Model file for the job. Use its own axes, mm. A direction names the side the tool comes from. Coordinates: 2 decimals unless noted, no trailing zeros. Order: outer loops, then holes, each group sorted by start corner. A loop starts at its lowest first (then second) coordinate and runs counter-clockwise, first axis right, second up. Notation, with made-up numbers: (-5.5, -1) - (41.5, -1) arc R4 ccw to (41.5, 4) - close; hole circle Ø4 at (-29.5, 50). An arc over 180 degrees is marked (long way). Put each result on its own line as item: value. Start each with the question number.
```python
from build123d import *

# Parameters (mm, degrees)
ESQUISSE2_R             = 6
BOSS_EXTRU_1_DEPTH      = 6
ESQUISSE3_R             = 3
BOSS_EXTRU_2_DEPTH      = 15.5
ESQUISSE4_W             = 12
ESQUISSE4_H             = 0.5
ENL_V_MAT_EXTRU_1_DEPTH = 7.75
ESQUISSE5_R             = 1.5
ENL_V_MAT_EXTRU_2_DEPTH = 3.5
ESQUISSE6_W             = 3
ESQUISSE6_H             = 1
BOSS_EXTRU_3_DEPTH      = 4
ESQUISSE7_R             = 18.5
BOSS_EXTRU_4_DEPTH      = 10
BOSS_EXTRU_4_DEPTH_BACK = 5


with BuildPart() as part:
    # Esquisse1 → Révolution1 (revolve)
    with BuildSketch(Plane.XY):
        Polygon((0, 0), (0, 7), (7, 7), (7, 16), (37, 16), (37, 18.5), (59, 18.5), (59, 0), align=None)
    revolve(axis=Axis((0, 0, 0), (1, 0, 0)))

    # Esquisse2 → Boss.-Extru.1 (add)
    with BuildSketch(Plane(origin=(59, 0, 0), x_dir=(0, 0, -1), z_dir=(1, 0, 0))):
        with Locations((0, 7)):
            Circle(ESQUISSE2_R)
    extrude(amount=BOSS_EXTRU_1_DEPTH)

    # Esquisse3 → Boss.-Extru.2 (add)
    with BuildSketch(Plane(origin=(65, 0, 0), x_dir=(0, 0, -1), z_dir=(1, 0, 0))):
        with Locations((0, 7)):
            Circle(ESQUISSE3_R)
    extrude(amount=BOSS_EXTRU_2_DEPTH)

    # Esquisse4 → Enlèv. mat.-Extru.1 (cut, symmetric)
    with BuildSketch(Plane.XY):
        with Locations((74.5, 4.25)):
            Rectangle(ESQUISSE4_W, ESQUISSE4_H)
    extrude(amount=ENL_V_MAT_EXTRU_1_DEPTH, both=True, mode=Mode.SUBTRACT)

    # Esquisse5 → Enlèv. mat.-Extru.2 (cut)
    with BuildSketch(Plane(origin=(59, 0, 0), x_dir=(0, 0, -1), z_dir=(1, 0, 0))):
        with Locations((15.5, 0)):
            Circle(ESQUISSE5_R)
        with Locations((7.75, 13.423393759)):
            Circle(ESQUISSE5_R)
        with Locations((7.75, -13.423393759)):
            Circle(ESQUISSE5_R)
        with Locations((-15.5, 0)):
            Circle(ESQUISSE5_R)
    extrude(amount=-ENL_V_MAT_EXTRU_2_DEPTH, mode=Mode.SUBTRACT)

    # Esquisse6 → Boss.-Extru.3 (add)
    with BuildSketch(Plane.ZY.offset(-7)):
        with Locations((0, 12.939057981)):
            Rectangle(ESQUISSE6_W, ESQUISSE6_H)
        with Locations((0, -12.939057981)):
            Rectangle(ESQUISSE6_W, ESQUISSE6_H)
    extrude(amount=BOSS_EXTRU_3_DEPTH)

    # Esquisse7 → Boss.-Extru.4 (add, two sides)
    with BuildSketch(Plane.ZY.offset(-7)) as boss_extru_4_sk:
        Circle(ESQUISSE7_R)
    extrude(amount=BOSS_EXTRU_4_DEPTH)
    extrude(boss_extru_4_sk.sketch, amount=-BOSS_EXTRU_4_DEPTH_BACK)


solid = part.part
```
Item 1: 3-axis set-ups, long thin cutter, end or side, ignore diameter. For faces 4 (the face through (12, 15, -6)), 5 (the face through (74, 4.5, 0)), 6 (the face through (57, 0, -14)), 7 (the face through (4.39, -18.06, -4.01)), 8 (the face through (-3, 0, 0)): which of +Z, -Z, +X, -X, +Y, -Y reach the whole face in a straight line?
Item 2: Slice it at C-C, the plane x = 23. Give the cut face in (y, z), plus the area to 3 significant figures.
Item 3: Slice it at D-D, the plane z = -7.75. Give the cut face in (x, y), plus the area to 3 significant figures.
Item 4: Slice it at A-A, the plane y = 0. Give the cut face in (x, z), plus the area to 3 significant figures.
Item 5: Flat gauge pins, fed straight in: pin 1 Ø2 at (x, y) = (47, -2) entering from +Z; pin 2 Ø5 at (x, y) = (5.5, -3.5) entering from -Z; pin 3 Ø12 at (x, y) = (55, -11) entering from -Z. Where does each tip first touch, or does it go through?
Item 6: Wall check: line 1 along Y through (x, z) = (57.75, -7.75); line 2 along X through (y, z) = (3, 15.5); line 3 along X through (y, z) = (7, 14.5). Give the ranges that are in metal, low to high.
Item 7: Pull direction Y, two halves, no side cores. Call faces 1 (the face through (24.68, -3.47, -15.62)), 2 (the face through (57.27, 11.96, -7.42)), 3 (the face through (80.5, 7, 0)): pulls with the +Y half, pulls with the -Y half, needs draft (parallel to the pull), parting line crosses it, or undercut.
Item 8: Slice it at B-B, the plane z = -4. Give the cut face in (x, y), plus the area to 3 significant figures.
Here are the results:
1. face 4: none
1. face 5: +Z, -Z, +X, -Y
1. face 6: +X
1. face 7: +X, -X
1. face 8: +Z, -Z, -X, +Y, -Y
2. outline: circle Ø32 at (0, 0)
2. area: 804 mm^2
3. outline: (-3, -16.8) - (12, -16.8) - (12, -14) - (37, -14) - (37, -16.8) - (59, -16.8) - (59, -14.92) - (55.5, -14.92) - (55.5, -11.92) - (59, -11.92) - (59, 11.92) - (55.5, 11.92) - (55.5, 14.92) - (59, 14.92) - (59, 16.8) - (37, 16.8) - (37, 14) - (12, 14) - (12, 16.8) - (-3, 16.8) - close
3. area: 1,920 mm^2
4. outline: (-3, -18.5) - (12, -18.5) - (12, -16) - (37, -16) - (37, -18.5) - (59, -18.5) - (59, -17) - (55.5, -17) - (55.5, -14) - (59, -14) - (59, 14) - (55.5, 14) - (55.5, 17) - (59, 17) - (59, 18.5) - (37, 18.5) - (37, 16) - (12, 16) - (12, 18.5) - (-3, 18.5) - close
4. area: 2,150 mm^2
5. pin 1: stops at z = 18.47
5. pin 2: stops at z = -18.47
5. pin 3: stops at z = -17.81
6. line 1: y = -16.8 to -14.92, -11.92 to 11.92, 14.92 to 16.8
6. line 2: x = -3 to 59
6. line 3: x = -3 to 12, 37 to 59
7. face 1: parting line crosses it
7. face 2: undercut
7. face 3: needs draft
8. outline: (-3, -18.06) - (12, -18.06) - (12, -15.49) - (37, -15.49) - (37, -18.06) - (59, -18.06) - (59, 2.53) - (65, 2.53) - (65, 11.47) - (59, 11.47) - (59, 18.06) - (37, 18.06) - (37, 15.49) - (12, 15.49) - (12, 18.06) - (-3, 18.06) - close
8. area: 2,160 mm^2
